Geometry: final body of the model. Coordinates: model frame, mm. Give positions to 0.01 mm unless a question says otherwise; leave off trailing zeros. Write each loop counter-clockwise with the first axis right and the second up, starting at its lowest first coordinate (ties: lowest second). Pieces come first, ordered by that corner, then holes.
from build123d import *

# Parameters (mm, degrees)
F3_W     = 127
F3_H     = 8.89
F4_DEPTH = 9.525
F5_W     = 133.35
F5_H     = 15.24
F6_DEPTH = 7.88512


with BuildPart() as f2:
    # F2: sweep along a path in F0
    with BuildLine(Plane.XY) as f2_path:
        Line((-63.5, 0), (63.5, 0))
        Line((63.5, 0), (63.5, -8.89))
        Line((63.5, -8.89), (-63.5, -8.89))
        Line((-63.5, -8.89), (-63.5, 0))
    # F1 (on Right) → F2 (sweep)
    with BuildSketch(Plane.YZ):
        with BuildLine():
            Line((0, 4.178553988), (0, 0))
            Line((0, 0), (15.875, 0))
            Line((15.875, 0), (15.875, 4.178553988))
            add(Edge.make_bspline(
                [(15.875, 4.178553988), (14.5700791907, 4.3410316154), (11.3910350226, 4.6434039972), (10.7282030423, 9.3279482792), (4.1216189564, 11.7033571608), (4.6891846979, 12.4869055891), (4.6625201725, 13.5694751074)],
                knots=[0, 0, 0, 0, 0.2552340564, 0.5197508028, 0.8294424133, 1, 1, 1, 1], degree=3))
            Line((4.6625201725, 13.5694751074), (2.7802032419, 13.5694751074))
            Line((2.7802032419, 13.5694751074), (2.7802032419, 15.875))
            Line((2.7802032419, 15.875), (0, 15.875))
            Line((0, 15.875), (0, 4.178553988))
        make_face()
    sweep(path=f2_path.line, transition=Transition.RIGHT)

    # F3 (on Top) → F4 (join)
    with BuildSketch(Plane.XY):
        with Locations((0, -4.445)):
            Rectangle(F3_W, F3_H)
    extrude(amount=F4_DEPTH)

    # F5 (on face) → F6 (cut)
    with BuildSketch(Plane(origin=(0, 0, 0), x_dir=(1, 0, 0), z_dir=(0, 0, -1))):
        with Locations((0, 4.445)):
            Rectangle(F5_W, F5_H)
    extrude(amount=-F6_DEPTH, mode=Mode.SUBTRACT)


solid = f2.part
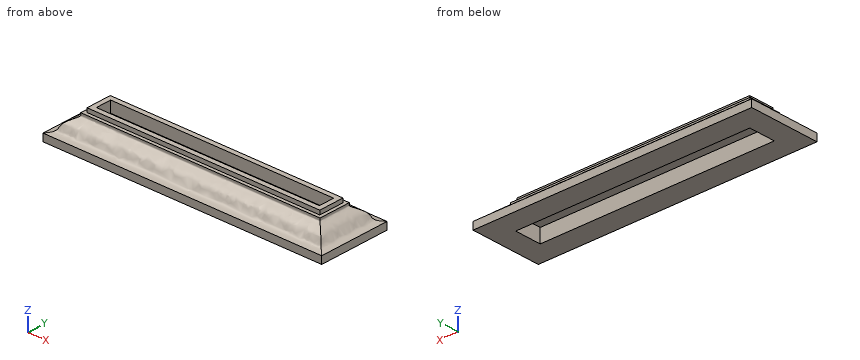
Q1. Pin query (flat end, axial travel): P1, Ø3, axis at x = -30.5, z = 11.5, coming from the +Y side; P2, Ø1.8, axis at y = -4, z = 14.5, coming from the +X side; P3, Ø1.2, axis at x = 0.5, z = 15, coming from the -Y side. Return the tip coordinate at first contact, or that it passes through.
Filled sheet:
P1: stops at y = 8.12
P2: stops at x = 66.28
P3: stops at y = -11.67
Q2. Ray query, line 1 along Y through (x, z) = (-57.5, 3) (3 decimals); line 2 along X through (y, z) = (-6, 13.25); line 3 along Y through (x, z) = (59, 12.5). Return the intervals inside material, ascending.
Filled sheet:
line 1: y = -24.765 to -12.065, 3.175 to 15.875
line 2: x = -68.16 to -63.5, 63.5 to 68.16
line 3: y = -13.53 to -8.89, 0 to 4.64
Q3. Section A-A on z = 2.75. Output: boundary loops of the cut face in (x, y) (3 decimals).
Filled sheet:
outline: (-79.375, -24.765) - (79.375, -24.765) - (79.375, 15.875) - (-79.375, 15.875) - close; hole (-66.675, -12.065) - (66.675, -12.065) - (66.675, 3.175) - (-66.675, 3.175) - close
